from build123d import *

# Parameters (mm, degrees)
SKETCH1_R           = 127
SKETCH1_R_2         = 3.175
BOSS_EXTRUDE1_DEPTH = 3.175


with BuildPart() as part:
    # Sketch1 → Boss-Extrude1 (new body)
    with BuildSketch(Plane(origin=(0, 0, 0), x_dir=(0, 0, -1), z_dir=(1, 0, 0))):
        Circle(SKETCH1_R)
        with BuildLine():
            ThreePointArc((-40.533501272, -58.531566299), (-34.11730778, -59.092910493), (-30.423072702, -64.368824956))
            Line((-30.423072702, -64.368824956), (-26.950595308, -84.062222874))
            ThreePointArc((-26.950595308, -84.062222874), (-29.658123464, -91.306232972), (-37.306264624, -92.451801739))
            ThreePointArc((-37.306264624, -92.451801739), (-49.8475, -86.33840263), (-61.412476619, -78.534073754))
            ThreePointArc((-61.412476619, -78.534073754), (-64.244455546, -71.337804834), (-59.324722854, -65.371011621))
            Line((-59.324722854, -65.371011621), (-40.533501272, -58.531566299))
        make_face(mode=Mode.SUBTRACT)
        with BuildLine():
            ThreePointArc((-70.956573975, 5.837258657), (-68.234615561, 0), (-70.956573975, -5.837258657))
            Line((-70.956573975, -5.837258657), (-86.275318162, -18.691211254))
            ThreePointArc((-86.275318162, -18.691211254), (-93.90257901, -19.968428138), (-98.718741244, -13.917727985))
            ThreePointArc((-98.718741244, -13.917727985), (-99.695, 0), (-98.718741244, 13.917727985))
            ThreePointArc((-98.718741244, 13.917727985), (-93.90257901, 19.968428138), (-86.275318162, 18.691211254))
            Line((-86.275318162, 18.691211254), (-70.956573975, 5.837258657))
        make_face(mode=Mode.SUBTRACT)
        with Locations((-29, -50.229473419)):
            Circle(SKETCH1_R_2, mode=Mode.SUBTRACT)
        with BuildLine():
            ThreePointArc((30.423072702, -64.368824956), (34.11730778, -59.092910493), (40.533501272, -58.531566299))
            Line((40.533501272, -58.531566299), (59.324722854, -65.371011621))
            ThreePointArc((59.324722854, -65.371011621), (64.244455546, -71.337804834), (61.412476619, -78.534073754))
            ThreePointArc((61.412476619, -78.534073754), (49.8475, -86.33840263), (37.306264624, -92.451801739))
            ThreePointArc((37.306264624, -92.451801739), (29.658123464, -91.306232972), (26.950595308, -84.062222874))
            Line((26.950595308, -84.062222874), (30.423072702, -64.368824956))
        make_face(mode=Mode.SUBTRACT)
        with Locations((29, -50.229473419)):
            Circle(SKETCH1_R_2, mode=Mode.SUBTRACT)
        with BuildLine():
            Line((16.085518962, 88.918512041), (23.091153482, 49.187584353))
            ThreePointArc((23.091153482, 49.187584353), (24.085087734, 46.788014801), (26, 45.033320997))
            ThreePointArc((26, 45.033320997), (28.477065544, 44.252305231), (31.05212086, 44.591317695))
            Line((31.05212086, 44.591317695), (68.962930813, 58.389724075))
            ThreePointArc((68.962930813, 58.389724075), (76.699872074, 58.693912553), (83.175501835, 54.449032119))
            ThreePointArc((83.175501835, 54.449032119), (86.33840263, 49.8475), (88.741995944, 44.807581502))
            ThreePointArc((88.741995944, 44.807581502), (89.180355355, 37.077081406), (85.048449775, 30.528787966))
            Line((85.048449775, 30.528787966), (54.143274342, 4.596266659))
            ThreePointArc((54.143274342, 4.596266659), (52.562153278, 2.53570957), (52, 0))
            ThreePointArc((52, 0), (52.562153278, -2.53570957), (54.143274342, -4.596266659))
            Line((54.143274342, -4.596266659), (85.048449775, -30.528787966))
            ThreePointArc((85.048449775, -30.528787966), (89.180355355, -37.077081406), (88.741995944, -44.807581502))
            ThreePointArc((88.741995944, -44.807581502), (86.33840263, -49.8475), (83.175501835, -54.449032119))
            ThreePointArc((83.175501835, -54.449032119), (76.699872074, -58.693912553), (68.962930813, -58.389724075))
            Line((68.962930813, -58.389724075), (31.05212086, -44.591317695))
            ThreePointArc((31.05212086, -44.591317695), (28.477065544, -44.252305231), (26, -45.033320997))
            ThreePointArc((26, -45.033320997), (24.085087734, -46.788014801), (23.091153482, -49.187584353))
            Line((23.091153482, -49.187584353), (16.085518962, -88.918512041))
            ThreePointArc((16.085518962, -88.918512041), (12.480483281, -95.770993959), (5.566494109, -99.256613621))
            ThreePointArc((5.566494109, -99.256613621), (0, -99.695), (-5.566494109, -99.256613621))
            ThreePointArc((-5.566494109, -99.256613621), (-12.480483281, -95.770993959), (-16.085518962, -88.918512041))
            Line((-16.085518962, -88.918512041), (-23.091153482, -49.187584353))
            ThreePointArc((-23.091153482, -49.187584353), (-24.085087734, -46.788014801), (-26, -45.033320997))
            ThreePointArc((-26, -45.033320997), (-28.477065544, -44.252305231), (-31.05212086, -44.591317695))
            Line((-31.05212086, -44.591317695), (-68.962930813, -58.389724075))
            ThreePointArc((-68.962930813, -58.389724075), (-76.699872074, -58.693912553), (-83.175501835, -54.449032119))
            ThreePointArc((-83.175501835, -54.449032119), (-86.33840263, -49.8475), (-88.741995944, -44.807581502))
            ThreePointArc((-88.741995944, -44.807581502), (-89.180355355, -37.077081406), (-85.048449775, -30.528787966))
            Line((-85.048449775, -30.528787966), (-54.143274342, -4.596266659))
            ThreePointArc((-54.143274342, -4.596266659), (-52.562153278, -2.53570957), (-52, 0))
            ThreePointArc((-52, 0), (-52.562153278, 2.53570957), (-54.143274342, 4.596266659))
            Line((-54.143274342, 4.596266659), (-85.048449775, 30.528787966))
            ThreePointArc((-85.048449775, 30.528787966), (-89.180355355, 37.077081406), (-88.741995944, 44.807581502))
            ThreePointArc((-88.741995944, 44.807581502), (-86.33840263, 49.8475), (-83.175501835, 54.449032119))
            ThreePointArc((-83.175501835, 54.449032119), (-76.699872074, 58.693912553), (-68.962930813, 58.389724075))
            Line((-68.962930813, 58.389724075), (-31.05212086, 44.591317695))
            ThreePointArc((-31.05212086, 44.591317695), (-28.477065544, 44.252305231), (-26, 45.033320997))
            ThreePointArc((-26, 45.033320997), (-24.085087734, 46.788014801), (-23.091153482, 49.187584353))
            Line((-23.091153482, 49.187584353), (-16.085518962, 88.918512041))
            ThreePointArc((-16.085518962, 88.918512041), (-12.480483281, 95.770993959), (-5.566494109, 99.256613621))
            ThreePointArc((-5.566494109, 99.256613621), (0, 99.695), (5.566494109, 99.256613621))
            ThreePointArc((5.566494109, 99.256613621), (12.480483281, 95.770993959), (16.085518962, 88.918512041))
        make_face(mode=Mode.SUBTRACT)
        with Locations((-58, 0)):
            Circle(SKETCH1_R_2, mode=Mode.SUBTRACT)
        with Locations((-29, 50.229473419)):
            Circle(SKETCH1_R_2, mode=Mode.SUBTRACT)
        with BuildLine():
            ThreePointArc((-30.423072702, 64.368824956), (-34.11730778, 59.092910493), (-40.533501272, 58.531566299))
            Line((-40.533501272, 58.531566299), (-59.324722854, 65.371011621))
            ThreePointArc((-59.324722854, 65.371011621), (-64.244455546, 71.337804834), (-61.412476619, 78.534073754))
            ThreePointArc((-61.412476619, 78.534073754), (-49.8475, 86.33840263), (-37.306264624, 92.451801739))
            ThreePointArc((-37.306264624, 92.451801739), (-29.658123464, 91.306232972), (-26.950595308, 84.062222874))
            Line((-26.950595308, 84.062222874), (-30.423072702, 64.368824956))
        make_face(mode=Mode.SUBTRACT)
        with Locations((58, 0)):
            Circle(SKETCH1_R_2, mode=Mode.SUBTRACT)
        with Locations((29, 50.229473419)):
            Circle(SKETCH1_R_2, mode=Mode.SUBTRACT)
        with BuildLine():
            ThreePointArc((70.956573975, -5.837258657), (68.234615561, 0), (70.956573975, 5.837258657))
            Line((70.956573975, 5.837258657), (86.275318162, 18.691211254))
            ThreePointArc((86.275318162, 18.691211254), (93.90257901, 19.968428138), (98.718741244, 13.917727985))
            ThreePointArc((98.718741244, 13.917727985), (99.695, 0), (98.718741244, -13.917727985))
            ThreePointArc((98.718741244, -13.917727985), (93.90257901, -19.968428138), (86.275318162, -18.691211254))
            Line((86.275318162, -18.691211254), (70.956573975, -5.837258657))
        make_face(mode=Mode.SUBTRACT)
        with BuildLine():
            ThreePointArc((40.533501272, 58.531566299), (34.11730778, 59.092910493), (30.423072702, 64.368824956))
            Line((30.423072702, 64.368824956), (26.950595308, 84.062222874))
            ThreePointArc((26.950595308, 84.062222874), (29.658123464, 91.306232972), (37.306264624, 92.451801739))
            ThreePointArc((37.306264624, 92.451801739), (49.8475, 86.33840263), (61.412476619, 78.534073754))
            ThreePointArc((61.412476619, 78.534073754), (64.244455546, 71.337804834), (59.324722854, 65.371011621))
            Line((59.324722854, 65.371011621), (40.533501272, 58.531566299))
        make_face(mode=Mode.SUBTRACT)
    extrude(amount=BOSS_EXTRUDE1_DEPTH)


solid = part.part
Verification items for the finished model (mm, model axes). Give positions to 0.01 mm unless a question says otherwise; leave off trailing zeros. Order: outer loops, then holes, each group sorted by start corner. A loop starts at its lowest first (then second) coordinate and runs counter-clockwise, first axis right, second up. Notation, with made-up numbers: (32, 30.5) -> (88, 30.5) arc R17 cw to (88, 34.5) -> close; hole circle Ø2 at (-4, 55.5). An arc over 180 degrees is marked (long way). Answer as CSV lines item,"result".
Q1. Release check for a two-part mould opening along Z. For faces 1 (the cylindrical face through (1.57, -123.98, 27.53)), 2 (the flat face through (1.565, 12.174, -78.509)), 3 (the cylindrical face through (1.57, 95.85, -12.4)), 4 (the flat face through (3.175, 2, -55)) record: +Z half, -Z half, draft (parallel to the pull), parting line (faces both ways), or undercut.
Solutions:
face 1,"parting line"
face 2,"undercut"
face 3,"undercut"
face 4,"draft"
Q2. Sectioned sample at B-B on y = 71. Record the cut outline in (x, z) (3 decimals).
Solutions:
outline,"(0, -105.3) -> (3.175, -105.3) -> (3.175, -64.183) -> (0, -64.183) -> close; (0, -29.254) -> (3.175, -29.254) -> (3.175, -19.245) -> (0, -19.245) -> close; (0, 19.245) -> (3.175, 19.245) -> (3.175, 29.254) -> (0, 29.254) -> close; (0, 64.183) -> (3.175, 64.183) -> (3.175, 105.3) -> (0, 105.3) -> close"
Q3. Scan lines: probe 1 along Y at (x, z) = (0.15, -74); probe 2 along Y at (x, z) = (0.7, -55.5); probe 3 along Y at (x, z) = (1.3, -35.5). Record each from-to range of solid material in increasing order.
Solutions:
probe 1,"y = -103.21 to -59.14, -21.26 to -8.39, 8.39 to 21.26, 59.14 to 103.21"
probe 2,"y = -114.23 to -82.82, -63.98 to -53.49, -5.73 to -1.96, 1.96 to 5.73, 53.49 to 63.98, 82.82 to 114.23"
probe 3,"y = -121.94 to -92.93, -58.47 to -46.21, 46.21 to 58.47, 92.93 to 121.94"
Q4. Sectioned sample at C-C on y = -24.5. Record the cut outline in (x, z) (3 decimals).
Solutions:
outline,"(0, -124.614) -> (3.175, -124.614) -> (3.175, -77.864) -> (0, -77.864) -> close; (0, 77.864) -> (3.175, 77.864) -> (3.175, 124.614) -> (0, 124.614) -> close"
Q5. Sectioned sample at A-A on z = 0. Record the cut outline in (x, y) (3 decimals).
Solutions:
outline,"(0, -127) -> (3.175, -127) -> (3.175, -99.695) -> (0, -99.695) -> close; (0, 99.695) -> (3.175, 99.695) -> (3.175, 127) -> (0, 127) -> close"
Q6. Depth check by flat-ended pin: pin 1 (1 mm diameter, centred on x = 1, y = -28.5, fed in from +Z); pin 2 (1.5 mm diameter, centred on x = 1.5, z = 37, fed in from -Y); pin 3 (5.5 mm diameter, centred on y = 0, z = 58, fed in from -X). Enter the tip coordinate at first touch or a pass-through.
Solutions:
pin 1,"stops at z = 123.87"
pin 2,"stops at y = -121.72"
pin 3,"passes through"
Q7. Sectioned sample at D-D on x = 1.05. Count the separate pieces of the cut face and the enclosed holes in it, plus the area to 3 significant figures.
Solutions:
separate pieces,"1"
enclosed holes,"13"
area,"25,900 mm²"
